Can you work these out from the model? Positions are in its coordinate system, mm. A direction names the side the tool comes from. Round coordinates to 2 decimals unless told otherwise and drop trailing zeros. Write each loop counter-clockwise with the first axis right and the second up, starting at its lowest first coordinate (ties: lowest second). Pieces come first, ordered by that corner, then holes.
Q1. We'd pull the mould along X, two halves only. Please class faces 1 (the flat face through (-4.59, -4.93, -6.04)), 2 (the flat face through (0, 0, 1)), 3 (the cylindrical face through (0.2, -4.9, 12.5)): +X half, -X half, draft (parallel to the pull), parting line (faces both ways), or undercut.
Q2. If we section it at B-B (x = -4.5): Please give me the cut outline in (y, z), plus the area to 3 significant figures.
Q3. If we section it at A-A (y = -9): Please give me the cut outline in (x, z).
Q4. I'm going to push flat-ended pins straight in: pin 1 Ø3 at (x, y) = (-1.5, -5) entering from -Z; pin 2 Ø1.5 at (y, z) = (-1.5, 7) entering from +X; pin 3 Ø2 at (x, y) = (4.5, -1.5) entering from -Z. Where does each tip first touch, or does it pass through?
Q5. Please list where these lines run through material, in increasing order: line 1 along X through (y, z) = (-4, -3); line 2 along Z through (x, y) = (-4, -6); line 3 along X through (y, z) = (-1.75, -7).
Q6. For faces 4 (the flat face through (0, -10, 1)), 5 (the flat face through (4.732, -4.93, -5.746)), which set-ups out of +Z, -Z, +X, -X, +Y, -Y let a thin tool reach every point of the face, with its end or its side?
from build123d import *

# Parameters (mm, degrees)
F0_R     = 12.5
F1_DEPTH = 10
F3_DEPTH = 25.4
F4_R     = 2


with BuildPart() as f1:
    # F0 (on Front) → F1 (new body)
    with BuildSketch(Plane.XZ):
        Circle(F0_R)
    extrude(amount=F1_DEPTH)

    # F2 (on face) → F3 (cut)
    with BuildSketch(Plane(origin=(0, 0, 0), x_dir=(-1, 0, 0), z_dir=(0, 1, 0))):
        with BuildLine():
            Line((0, 0), (-7.94716, -9.648453))
            ThreePointArc((-7.94716, -9.648453), (-0.243247, -12.497633), (7.565699, -9.950387))
            Line((7.565699, -9.950387), (0, 0))
        make_face()
    extrude(amount=-F3_DEPTH, mode=Mode.SUBTRACT)

    # F4
    f4_edges = [f1.edges().sort_by_distance(p)[0] for p in [
        (0, -5, 0),
    ]]
    fillet(f4_edges, radius=F4_R)


solid = f1.part
A:
1. face 1: undercut
1. face 2: draft
1. face 3: parting line
2. outline: (-10, -5.92) - (0, -5.92) - (0, 11.66) - (-10, 11.66) - close
2. area: 176 mm2
3. outline: (-7.57, -9.95) - (-1.53, -2.01) arc R2 cw to (1.61, -1.95) - (7.95, -9.65) arc R12.5 ccw (long way) to start
4. pin 1: stops at z = -3.95
4. pin 2: stops at x = 10.83
4. pin 3: stops at z = -6.68
5. line 1: x = -12.13 to -2.28, 2.47 to 12.13
5. line 2: z = -5.26 to 11.84
5. line 3: x = -10.36 to -5.32, 5.77 to 10.36
6. face 4: +Z, -Z, +X, -X, -Y
6. face 5: -Z, +Y, -Y
